Input: part model. Units: mm. Frame: model coordinates. A direction names the side the tool comes from. Give positions to 0.01 mm unless a question says otherwise; leave off trailing zeros. Loops run counter-clockwise (first coordinate to the right, second up) from the corner with the lowest first, then second, coordinate; pieces in that order, holes last.
from build123d import *

# Parameters (mm, degrees)
F0_W     = 5.08
F0_H     = 55.245
F1_DEPTH = 184.15
F2_R     = 6.35
F3_DEPTH = 25.4
F4_R     = 6.35
F5_DEPTH = 25.4


with BuildPart() as f1:
    # F0 (on Front) → F1 (new body)
    with BuildSketch(Plane.XZ):
        Polygon((26.67, 0), (0, 0), (-5.08, 0), (-5.08, -5.08), (26.67, -5.08), align=None)
        with Locations((-2.54, 27.6225)):
            Rectangle(F0_W, F0_H)
    extrude(amount=F1_DEPTH)

    # F2 (on face) → F3 (cut)
    with BuildSketch(Plane.YZ):
        with Locations((-149.225, 45.72)):
            Circle(F2_R)
        with Locations((-34.925, 45.72)):
            Circle(F2_R)
    extrude(amount=-F3_DEPTH, mode=Mode.SUBTRACT)

    # F4 (on face) → F5 (cut)
    with BuildSketch(Plane.XY):
        with Locations((11.7475, -149.225)):
            Circle(F4_R)
        with Locations((11.7475, -34.925)):
            Circle(F4_R)
    extrude(amount=-F5_DEPTH, mode=Mode.SUBTRACT)


solid = f1.part
(1) Mould query, pull axis Y, two halves, no side actions, for faces 1 (the flat face through (-1, 0, 19)), 2 (the flat face through (26.67, -91, -3)), 3 (the cylindrical face through (7.1, -144.9, -2.5)). Classes: +Y half, -Y half, draft (parallel to the pull), parting line (faces both ways), or undercut.
Values follow:
face 1: +Y half
face 2: draft
face 3: undercut
(2) Cut plane B-B (x = 13). Return the cut outline in (y, z).
Values follow:
outline: (-184.15, -5.08) - (-155.45, -5.08) - (-155.45, 0) - (-184.15, 0) - close; (-143, -5.08) - (-41.15, -5.08) - (-41.15, 0) - (-143, 0) - close; (-28.7, -5.08) - (0, -5.08) - (0, 0) - (-28.7, 0) - close
(3) Cut plane A-A (z = 45.72). Return the cut outline in (x, y) (3 decimals), and give its area (3 significant figures).
Values follow:
outline: (-5.08, -184.15) - (0, -184.15) - (0, -155.575) - (-5.08, -155.575) - close; (-5.08, -142.875) - (0, -142.875) - (0, -41.275) - (-5.08, -41.275) - close; (-5.08, -28.575) - (0, -28.575) - (0, 0) - (-5.08, 0) - close
area: 806 mm2
(4) Cut plane C-C (y = -73). Return the cut outline in (x, z) (3 decimals).
Values follow:
outline: (-5.08, -5.08) - (26.67, -5.08) - (26.67, 0) - (0, 0) - (0, 55.245) - (-5.08, 55.245) - close
(5) Ray query, probe 1 along Z at (x, y) = (16.5, -162); probe 2 along Z at (x, y) = (-1.5, -36) (3 decimals). Return the intervals inside material, ascending.
Values follow:
probe 1: z = -5.08 to 0
probe 2: z = -5.08 to 39.462, 51.978 to 55.245
(6) Cut plane D-D (z = 35.5). Return the cut outline in (x, y), and give its area (3 significant figures).
Values follow:
outline: (-5.08, -184.15) - (0, -184.15) - (0, 0) - (-5.08, 0) - close
area: 935 mm2
(7) Reachability of faces 4 (the flat face through (0, -91, 27)), 5 (the cylindrical face through (6.71, -38.79, -2.5)) from +Z, -Z, +X, -X, +Y, -Y: full face, straight path, thin tool, end or side. Return the list, or none.
Values follow:
face 4: +Z, +X, +Y, -Y
face 5: +Z, -Z
(8) Pin query (flat end, axial travel): pin 1 Ø16.5 at (y, z) = (-108.5, 21) entering from +X; pin 2 Ø2 at (x, y) = (10.5, -112) entering from +Z. Return the tip coordinate at first contact, or that it passes through.
Values follow:
pin 1: stops at x = 0
pin 2: stops at z = 0
